CAD build for the part. Positions are in the model's coordinates, mm. A direction names the side the tool comes from. Give positions to 0.01 mm unless a question says otherwise; leave off trailing zeros. Loops run counter-clockwise (first coordinate to the right, second up) from the corner with the lowest first, then second, coordinate; pieces in that order, holes last.
Item 1: Mould opens along X. For faces 1 (the flat face through (60.452, -1, -1)), 2 (the flat face through (-1.436, -1, -59)), 3 (the flat face through (13, -1, 63.5)) say: released by +X, released by -X, zero draft, split by the parting line, or undercut.
Item 2: Drop flat-ended pins along their axis: P1, Ø0.5, axis at x = 2, y = -1.5, coming from the +Z side; P2, Ø0.8, axis at x = 2.5, y = -2, coming from the -Z side. Give the stop position or say it passes through.
Item 3: Probe probe 1 along X at (y, z) = (-1.75, 58); probe 2 along Z at (x, y) = (-3, -2.4); probe 3 along Z at (x, y) = (35, -1.7). List the from-to ranges inside material, lowest first.
Item 4: Which spindle directions (+Z, -Z, +X, -X, +Y, -Y) get a long thin tool onto all of the face, cutting with end or side? Do faces 4 (the flat face through (30.162, -1, 59)), 5 (the flat face through (54, -1, -63.5)), 6 (the flat face through (30.162, -1, -52)). Say none if no direction does.
Item 5: Saw through at A-A on z = -52. Give the cut face in (x, y), plus the area to 3 significant figures.
Item 6: Saw through at B-B on x = -40. Give the cut face in (y, z).
from build123d import *

# Parameters (mm, degrees)
F1_DEPTH = 2.9718


with BuildPart() as f1:
    # F0 (on Front) → F1 (new body)
    with BuildSketch(Plane.XZ):
        Polygon((-63.5, -60.452), (-63.5, -63.5), (-47.625, -63.5), (-47.625, -60.452), (-33.274, -60.452), (-33.274, -56.642), (-34.925, -56.642), (-34.925, -54.26075), (-33.274, -54.26075), (-33.274, -50.292), (-31.75, -50.292), (-30.226, -50.292), (-30.226, -54.26075), (-28.575, -54.26075), (-28.575, -56.642), (-30.226, -56.642), (-30.226, -60.452), (-15.875, -60.452), (-15.875, -63.5), (-9.525, -63.5), (-9.525, -60.452), (-1.436332, -60.452), (-1.436332, -56.642), (-3.087332, -56.642), (-3.087332, -54.26075), (-1.436332, -54.26075), (-1.436332, -50.292), (0.087668, -50.292), (1.611668, -50.292), (1.611668, -54.26075), (3.262668, -54.26075), (3.262668, -56.642), (1.611668, -56.642), (1.611668, -60.452), (9.525, -60.452), (9.525, -63.5), (15.875, -63.5), (15.875, -60.452), (30.1625, -60.452), (30.1625, -56.642), (28.575, -56.642), (28.575, -54.26075), (30.1625, -54.26075), (30.1625, -50.292), (31.75, -50.292), (33.3375, -50.292), (33.3375, -54.26075), (34.925, -54.26075), (34.925, -56.642), (33.3375, -56.642), (33.3375, -60.452), (47.625, -60.452), (47.625, -63.5), (60.452, -63.5), (60.452, 0), (-63.5, 0), align=None)
        Polygon((-63.5, 60.452), (-63.5, 0), (60.452, 0), (60.452, 63.5), (47.625, 63.5), (47.625, 60.452), (33.3375, 60.452), (33.3375, 56.642), (34.925, 56.642), (34.925, 54.26075), (33.3375, 54.26075), (33.3375, 50.292), (31.75, 50.292), (30.1625, 50.292), (30.1625, 54.26075), (28.575, 54.26075), (28.575, 56.642), (30.1625, 56.642), (30.1625, 60.452), (15.875, 60.452), (15.875, 63.5), (9.525, 63.5), (9.525, 60.452), (1.611668, 60.452), (1.611668, 56.642), (3.262668, 56.642), (3.262668, 54.26075), (1.611668, 54.26075), (1.611668, 50.292), (0.087668, 50.292), (-1.436332, 50.292), (-1.436332, 54.26075), (-3.087332, 54.26075), (-3.087332, 56.642), (-1.436332, 56.642), (-1.436332, 60.452), (-9.525, 60.452), (-9.525, 63.5), (-15.875, 63.5), (-15.875, 60.452), (-30.226, 60.452), (-30.226, 56.642), (-28.575, 56.642), (-28.575, 54.26075), (-30.226, 54.26075), (-30.226, 50.292), (-31.75, 50.292), (-33.274, 50.292), (-33.274, 54.26075), (-34.925, 54.26075), (-34.925, 56.642), (-33.274, 56.642), (-33.274, 60.452), (-47.625, 60.452), (-47.625, 63.5), (-63.5, 63.5), align=None)
    extrude(amount=F1_DEPTH)


solid = f1.part
Results below:
1. face 1: released by +X
1. face 2: undercut
1. face 3: zero draft
2. P1: stops at z = 60.45
2. P2: stops at z = -60.45
3. probe 1: x = -63.5 to -33.27, -30.23 to -1.44, 1.61 to 30.16, 33.34 to 60.45
3. probe 2: z = -60.45 to -56.64, -54.26 to 54.26, 56.64 to 60.45
3. probe 3: z = -60.45 to 60.45
4. face 4: +Z, +Y, -Y
4. face 5: -Z, +X, -X, +Y, -Y
4. face 6: -Z, +Y, -Y
5. outline: (-63.5, -2.97) - (-33.27, -2.97) - (-33.27, 0) - (-63.5, 0) - close; (-30.23, -2.97) - (-1.44, -2.97) - (-1.44, 0) - (-30.23, 0) - close; (1.61, -2.97) - (30.16, -2.97) - (30.16, 0) - (1.61, 0) - close; (33.34, -2.97) - (60.45, -2.97) - (60.45, 0) - (33.34, 0) - close
5. area: 341 mm2
6. outline: (-2.97, -60.45) - (0, -60.45) - (0, 60.45) - (-2.97, 60.45) - close
